Study the drawing (mm; zero at the part's minimum x, y, z) and answer. A direction names the side the tool comes from. Give positions to 0.01 mm unless a question says otherwise; leave off trailing zeros. Order: outer loops, then holes, each group sorted by start corner. A loop starts at its lowest first (then second) coordinate and runs counter-clockwise, first axis right, second up. Notation, with made-up numbers: (18.25, -9.75) - (24.25, -9.75) arc R24 ccw to (24.25, 27.25) - close; hole circle Ø6 at (-12.5, 9.25). An arc over 180 degrees is marked (long way). Write each question's results on one line, items separated by ' | '. Start each with the question number.
1. Flat-ended cylindrical pins translate along their axes: pin 1 (1.5 mm diameter, centred on x = 20, y = 9, fed in from -Z); pin 2 (4.5 mm diameter, centred on y = 23.5, z = 10.97, fed in from +X); pin 3 (1.5 mm diameter, centred on x = 20, y = 5, fed in from +Z). Find the tip coordinate at first contact, or state that the pin passes through.
2. Find the intervals of material crossed by L1, parallel to Y at x = 39.2, z = 10.97; L2, parallel to Y at x = 20, z = 39.25; L3, parallel to X at y = 23, z = 24 (3 decimals), in increasing order.
3. Which of the six approach directions +Z, -Z, +X, -X, +Y, -Y give full straight-line access (tool end or side, diameter ignored) to the marked faces 4 and 5?
4. Section A-A (z = 28.5) is taken. Give the vertices of the cut face in (x, y) (3 decimals), and give its area (3 significant figures).
5. Determine the mould class of the marked faces 1, 2 and 3 for opening direction X: released by +X, released by -X, zero draft, split by the parting line, or undercut.
6. Section B-B (y = 15.5) is taken. Give the vertices of the cut face in (x, z) (3 decimals), and give its area (3 significant figures).
7. Section D-D (y = 7.5) is taken. Give the vertices of the cut face in (x, z) (3 decimals), and give its area (3 significant figures).
8. Section C-C (x = 20) is taken. Give the vertices of the cut face in (y, z), and give its area (3 significant figures).
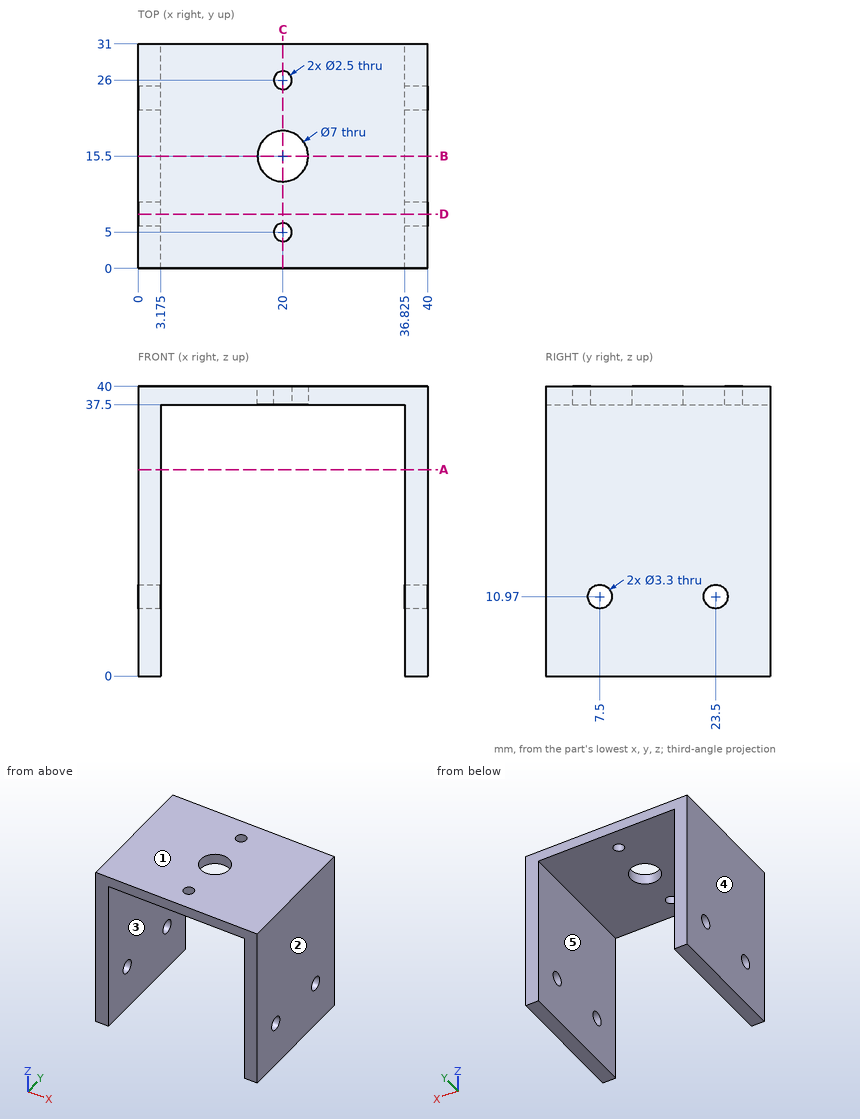
Reported:
1) pin 1: z = 37.5 | pin 2: x = 40 | pin 3: through
2) L1: 0 to 5.85, 9.15 to 21.85, 25.15 to 31 | L2: 0 to 3.75, 6.25 to 12, 19 to 24.75, 27.25 to 31 | L3: 0 to 3.175, 36.825 to 40
3) face 4: +Z, -Z, -X, +Y, -Y | face 5: -Z, +Y, -Y
4) outline: (0, 0) - (3.175, 0) - (3.175, 31) - (0, 31) - close; (36.825, 0) - (40, 0) - (40, 31) - (36.825, 31) - close | area: 197 mm²
5) face 1: zero draft | face 2: released by +X | face 3: undercut
6) outline: (0, 0) - (3.175, 0) - (3.175, 37.5) - (16.5, 37.5) - (16.5, 40) - (0, 40) - close; (23.5, 37.5) - (36.825, 37.5) - (36.825, 0) - (40, 0) - (40, 40) - (23.5, 40) - close | area: 321 mm²
7) outline: (0, 0) - (3.175, 0) - (3.175, 9.32) - (0, 9.32) - close; (0, 12.62) - (3.175, 12.62) - (3.175, 37.5) - (36.825, 37.5) - (36.825, 12.62) - (40, 12.62) - (40, 40) - (0, 40) - close; (36.825, 0) - (40, 0) - (40, 9.32) - (36.825, 9.32) - close | area: 317 mm²
8) outline: (0, 37.5) - (3.75, 37.5) - (3.75, 40) - (0, 40) - close; (6.25, 37.5) - (12, 37.5) - (12, 40) - (6.25, 40) - close; (19, 37.5) - (24.75, 37.5) - (24.75, 40) - (19, 40) - close; (27.25, 37.5) - (31, 37.5) - (31, 40) - (27.25, 40) - close | area: 47.5 mm²
